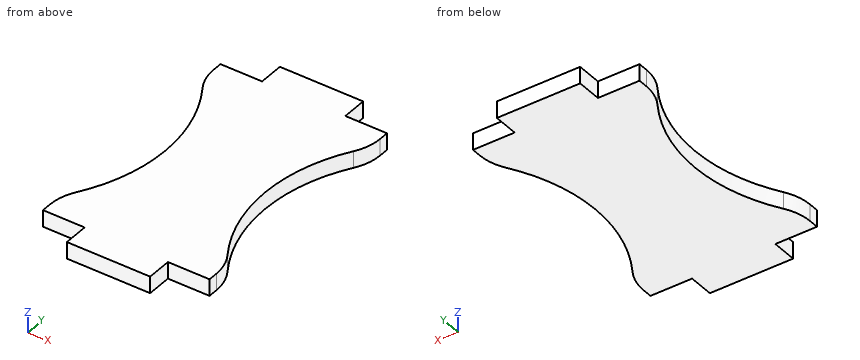
```python
from build123d import *

# Parameters (mm, degrees)
EXTRUDE_1_DEPTH = 2


with BuildPart() as part:
    # Model → Бобышка-Вытянуть1 (new body)
    with BuildSketch(Plane.XY):
        with BuildLine():
            Line((-10, 33), (-5, 33))
            Line((-5, 33), (-5, 36))
            Line((-5, 36), (5, 36))
            Line((5, 36), (5, 33))
            Line((5, 33), (10, 33))
            Line((10, 33), (10, 31.856406461))
            ThreePointArc((10, 31.856406461), (9.764613537, 30.192305872), (9.076923077, 28.6587742))
            ThreePointArc((9.076923077, 28.6587742), (6, 18), (9.076923077, 7.3412258))
            ThreePointArc((9.076923077, 7.3412258), (9.764613537, 5.807694128), (10, 4.143593539))
            Line((10, 4.143593539), (10, 3))
            Line((10, 3), (5, 3))
            Line((5, 3), (5, 0))
            Line((5, 0), (-5, 0))
            Line((-5, 0), (-5, 3))
            Line((-5, 3), (-10, 3))
            Line((-10, 3), (-10, 4.143593539))
            ThreePointArc((-10, 4.143593539), (-9.764613537, 5.807694128), (-9.076923077, 7.3412258))
            ThreePointArc((-9.076923077, 7.3412258), (-6.000000001, 18), (-9.076923078, 28.6587742))
            ThreePointArc((-9.076923078, 28.6587742), (-9.764613538, 30.192305872), (-10, 31.856406461))
            Line((-10, 31.856406461), (-10, 33))
        make_face()
    extrude(amount=EXTRUDE_1_DEPTH)


solid = part.part
```
Input: part model. Units: mm. Frame: model coordinates. Give positions to 0.01 mm unless a question says otherwise; leave off trailing zeros. Write each loop counter-clockwise with the first axis right and the second up, starting at its lowest first coordinate (ties: lowest second). Pieces come first, ordered by that corner, then holes. Notation, with made-up numbers: (78.5, 61) - (136.5, 61) arc R28 cw to (136.5, 92) - close; hole circle Ø9 at (-13, 76.25). An arc over 180 degrees is marked (long way). Write item = value, one per line. Start each with the question number.
1. First-contact query: pin 1 Ø0.6 at (y, z) = (1.5, 0.5) entering from +X; pin 2 Ø1 at (x, z) = (-7, 0.5) entering from -Y. Flat tips, straight axial feed; report the tip coordinate or a pass-through.
2. Section query B-B, the plane x = -5.5. Output: boundary loops of the cut face in (y, z).
3. Ray query, L1, parallel to X at y = 34, z = 1.75; L2, parallel to Y at x = 8.75, z = 0.6; L3, parallel to Y at x = -7.75, z = 0.25. Return the intervals inside material, ascending.
4. Section query C-C, the plane y = 20.5. Output: boundary loops of the cut face in (x, z).
5. Section query A-A, the plane z = 1.55. Output: boundary loops of the cut face in (x, y).
Check sheet entries:
q1.pin_1 = 5
q1.pin_2 = 3
q2.outline = (3, 0) - (33, 0) - (33, 2) - (3, 2) - close
q3.L1 = -5 to 5
q3.L2 = 3 to 7.88, 28.12 to 33
q3.L3 = 3 to 9.82, 26.18 to 33
q4.outline = (-6.16, 0) - (6.16, 0) - (6.16, 2) - (-6.16, 2) - close
q5.outline = (-10, 3) - (-5, 3) - (-5, 0) - (5, 0) - (5, 3) - (10, 3) - (10, 4.14) arc R6 ccw to (9.08, 7.34) arc R20 cw to (9.08, 28.66) arc R6 ccw to (10, 31.86) - (10, 33) - (5, 33) - (5, 36) - (-5, 36) - (-5, 33) - (-10, 33) - (-10, 31.86) arc R6 ccw to (-9.08, 28.66) arc R20 cw to (-9.08, 7.34) arc R6 ccw to (-10, 4.14) - close
